Geometry check sheet. Reference: the model listing, model coordinates, mm. A direction names the side the tool comes from. Give positions to 0.01 mm unless a question says otherwise; leave off trailing zeros. Loops run counter-clockwise (first coordinate to the right, second up) from the corner with the lowest first, then second, coordinate; pieces in that order, holes last. Notation, with made-up numbers: (-22, 55.5) -> (29, 55.5) arc R20 ccw to (29, 75.5) -> close; hole circle Ø6 at (-32, 39). An arc over 180 degrees is marked (long way). One line per item, written item: value. Start each with the question number.
(1) Gauge pin test, flat ends, axial feed: pin 1 Ø3 at (y, z) = (4.5, 0) entering from -X; pin 2 Ø8 at (x, y) = (-1, 7) entering from -Z; pin 3 Ø12 at (y, z) = (4, -12) entering from -X; pin 4 Ø4 at (y, z) = (8.75, 0) entering from +X. Record the tip position at first contact, or that the pin passes through.
(2) Draft check along X on faces 1 (the face through (-0.1, 0.8, 3)), 2 (the face through (0, -4, 0)), 3 (the face through (36, 13, -7)), 4 (the face through (-11, 6, 0)). Enter one of: pulls with the +X half, pulls with the -X half, needs draft (parallel to the pull), parting line crosses it, or undercut.
(3) Scan lines: line 1 along Y through (x, z) = (-12.55, 0); line 2 along Y through (x, z) = (-15.5, -1). Record each from-to range of solid material in increasing order. Write a range as from..to.
(4) Sectioned sample at B-B, the plane y = -8.75. Record the cut outline in (x, z), then the cut area to 3 significant figures.
(5) Sectioned sample at A-A, the plane x = 1.5. Record the cut outline in (y, z).
(6) Sectioned sample at C-C, the plane y = -5.5. Record the cut outline in (x, z), then the cut area to 3 significant figures.
(7) Sectioned sample at D-D, the plane z = 0. State how many separate pieces and enclosed holes the cut face has, then the cut area to 4 significant figures.
(8) Tool access check on faces 5 (the face through (-13, -11.75, 0)), 6 (the face through (-14, 0, 0)), 7 (the face through (-0.1, 0.8, -3)). Record the directions out of +Z, -Z, +X, -X, +Y, -Y that give a thin tool (end or side, any length) a straight path to the whole face; none if there is none.
from build123d import *

# Parameters (mm, degrees)
SALIENTE_EXTRUIR1_DEPTH      = 14
CROQUIS3_W                   = 6
CROQUIS3_H                   = 23.5
CROQUIS3_R                   = 1.75
SALIENTE_EXTRUIR2_DEPTH      = 3
REDONDEO1_R                  = 2
REDONDEO1_OF_SIMETR_A1_R     = 2
CROQUIS6_W                   = 72
CROQUIS6_H                   = 27.119895789
SALIENTE_EXTRUIR5_DEPTH      = 2
SALIENTE_EXTRUIR5_DEPTH_BACK = 0.25


with BuildPart() as part:
    # Croquis2 → Saliente-Extruir1 (new body)
    with BuildSketch(Plane(origin=(0, 0, 0), x_dir=(0, 0, -1), z_dir=(1, 0, 0))):
        with BuildLine():
            Line((-3, -1), (-3, 1))
            ThreePointArc((-3, 1), (0, 4), (3, 1))
            Line((3, 1), (3, -1))
            ThreePointArc((3, -1), (0, -4), (-3, -1))
        make_face()
    saliente_extruir1 = extrude(amount=SALIENTE_EXTRUIR1_DEPTH)

    # Croquis3 → Saliente-Extruir2 (add)
    with BuildSketch(Plane(origin=(14, 0, 0), x_dir=(0, 0, -1), z_dir=(1, 0, 0))):
        Rectangle(CROQUIS3_W, CROQUIS3_H)
        with Locations((0, 8.75)):
            Circle(CROQUIS3_R, mode=Mode.SUBTRACT)
        with Locations((0, -8.75)):
            Circle(CROQUIS3_R, mode=Mode.SUBTRACT)
    saliente_extruir2 = extrude(amount=-SALIENTE_EXTRUIR2_DEPTH)

    # Redondeo1
    redondeo1_edges = [part.edges().sort_by_distance(p)[0] for p in [
        (12.5, -11.75, -3),
        (12.5, -11.75, 3),
    ]]
    fillet(redondeo1_edges, radius=REDONDEO1_R)

    # Simetría1: Saliente-Extruir1, Saliente-Extruir2 across plane
    add(saliente_extruir1.mirror(Plane(origin=(0, 0, 0), x_dir=(0, 0, 1), z_dir=(1, 0, 0))))
    add(saliente_extruir2.mirror(Plane(origin=(0, 0, 0), x_dir=(0, 0, 1), z_dir=(1, 0, 0))))

    # Redondeo1 of Simetría1
    redondeo1_of_simetr_a1_edges = [part.edges().sort_by_distance(p)[0] for p in [
        (-12.5, -11.75, -3),
        (-12.5, -11.75, 3),
    ]]
    fillet(redondeo1_of_simetr_a1_edges, radius=REDONDEO1_OF_SIMETR_A1_R)

    # Croquis6 → Saliente-Extruir5 (add, two sides)
    with BuildSketch(Plane(origin=(0, 11.75, 0), x_dir=(1, 0, 0), z_dir=(0, 1, 0))) as saliente_extruir5_sk:
        with Locations((0, 7.059947895)):
            Rectangle(CROQUIS6_W, CROQUIS6_H)
    extrude(amount=SALIENTE_EXTRUIR5_DEPTH)
    extrude(saliente_extruir5_sk.sketch, amount=-SALIENTE_EXTRUIR5_DEPTH_BACK)


solid = part.part
Calculated:
1. pin 1: stops at x = -14
1. pin 2: stops at z = -2.24
1. pin 3: passes through
1. pin 4: stops at x = 14
2. face 1: needs draft
2. face 2: undercut
2. face 3: pulls with the +X half
2. face 4: undercut
3. line 1: y = -11.75..-10.5, -7..7, 10.5..13.75
3. line 2: y = 11.5..13.75
4. outline: (-14, -3) -> (-11, -3) -> (-11, -1.75) -> (-14, -1.75) -> close; (-14, 1.75) -> (-11, 1.75) -> (-11, 3) -> (-14, 3) -> close; (11, -3) -> (14, -3) -> (14, -1.75) -> (11, -1.75) -> close; (11, 1.75) -> (14, 1.75) -> (14, 3) -> (11, 3) -> close
4. area: 15.0 mm2
5. outline: (-1, -3) -> (1, -3) arc R3 ccw to (1, 3) -> (-1, 3) arc R3 ccw to start; (11.5, -20.62) -> (13.75, -20.62) -> (13.75, 6.5) -> (11.5, 6.5) -> close
6. outline: (-14, -3) -> (-11, -3) -> (-11, 3) -> (-14, 3) -> close; (11, -3) -> (14, -3) -> (14, 3) -> (11, 3) -> close
6. area: 36.0 mm2
7. separate pieces: 4
7. enclosed holes: 0
7. area: 435.5 mm2
8. face 5: +Z, -Z, +X, -X, -Y
8. face 6: +Z, -Z, -X, -Y
8. face 7: -Z, +X, -X, -Y
